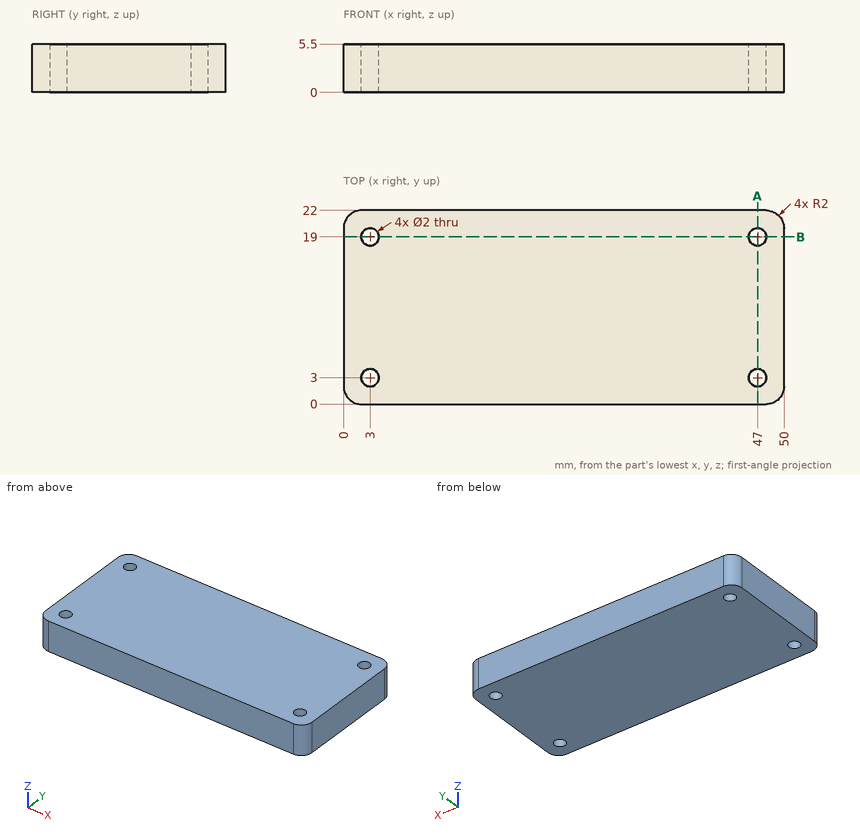
For this review, use the dimensioned drawing (mm, ordinates from the lowest corner) and the shaded views. Round coordinates to 2 decimals unless told otherwise and drop trailing zeros. Write each loop counter-clockwise with the first axis right and the second up, starting at its lowest first coordinate (ties: lowest second). Pieces come first, ordered by that corner, then holes. Notation, with made-up numbers: (31.25, 54.5) - (60.25, 54.5) arc R30 ccw to (60.25, 89.5) - close; hole circle Ø2 at (-21.75, 38.25). An arc over 180 degrees is marked (long way). Answer as CSV lines item,"result". Start each with the question number.
(1) We need section B-B on y = 19. State the section outline as (x, z) points.
(2) We need section A-A on x = 47. State the section outline as (y, z) points.
(3) To check wall thickness, follow line 1 (X direction, y = 3, z = 1.7); line 2 (Y direction, x = 3, z = 1.15); line 3 (X direction, y = 20.5, z = 1.6). State the ranges of each line that lie inside material, in increasing order.
Worked answers:
1,outline,"(0, 0) - (2, 0) - (2, 5.5) - (0, 5.5) - close; (4, 0) - (46, 0) - (46, 5.5) - (4, 5.5) - close; (48, 0) - (50, 0) - (50, 5.5) - (48, 5.5) - close"
2,outline,"(0, 0) - (2, 0) - (2, 5.5) - (0, 5.5) - close; (4, 0) - (18, 0) - (18, 5.5) - (4, 5.5) - close; (20, 0) - (22, 0) - (22, 5.5) - (20, 5.5) - close"
3,line 1,"0 to 2, 4 to 46, 48 to 50"
3,line 2,"0 to 2, 4 to 18, 20 to 22"
3,line 3,"0.06 to 49.94"
